```python
from build123d import *

# Parameters (mm, degrees)
SCHIZZO1_R                   = 14
ESTRUSIONE_ESTRUSIONE1_DEPTH = 40
SCHIZZO4_R                   = 2
TAGLIO_ESTRUSIONE1_DEPTH     = 10
SCHIZZO5_R                   = 2
TAGLIO_ESTRUSIONE2_DEPTH     = 10
SCHIZZO6_W                   = 32.003306677
SCHIZZO6_H                   = 7.880991961
TAGLIO_ESTRUSIONE3_DEPTH     = 20


with BuildPart() as part:
    # Schizzo1 → Estrusione-Estrusione1 (new body)
    with BuildSketch(Plane.XY):
        with BuildLine():
            Line((20, -13.266499161), (20, 13.266499161))
            ThreePointArc((20, 13.266499161), (0, 24), (-20, 13.266499161))
            Line((-20, 13.266499161), (-20, -13.266499161))
            ThreePointArc((-20, -13.266499161), (0, -24), (20, -13.266499161))
        make_face()
        Circle(SCHIZZO1_R, mode=Mode.SUBTRACT)
    extrude(amount=-ESTRUSIONE_ESTRUSIONE1_DEPTH)

    # Schizzo4 → Taglio-Estrusione1 (cut)
    with BuildSketch(Plane.ZY.offset(20)):
        with Locations((-10, 10)):
            Circle(SCHIZZO4_R)
        with Locations((-10, -10)):
            Circle(SCHIZZO4_R)
        with Locations((-30, -10)):
            Circle(SCHIZZO4_R)
        with Locations((-30, 10)):
            Circle(SCHIZZO4_R)
    extrude(amount=-TAGLIO_ESTRUSIONE1_DEPTH, mode=Mode.SUBTRACT)

    # Schizzo5 → Taglio-Estrusione2 (cut)
    with BuildSketch(Plane.XY):
        with Locations((-13.435028843, 13.435028843)):
            Circle(SCHIZZO5_R)
        with Locations((13.435028843, 13.435028843)):
            Circle(SCHIZZO5_R)
        with Locations((13.435028843, -13.435028843)):
            Circle(SCHIZZO5_R)
        with Locations((-13.435028843, -13.435028843)):
            Circle(SCHIZZO5_R)
    extrude(amount=-TAGLIO_ESTRUSIONE2_DEPTH, mode=Mode.SUBTRACT)

    # Schizzo6 → Taglio-Estrusione3 (cut)
    with BuildSketch(Plane(origin=(0, 0, -40), x_dir=(-1, 0, 0), z_dir=(0, 0, -1))):
        with Locations((0.127145472, 21.940495981)):
            Rectangle(SCHIZZO6_W, SCHIZZO6_H)
        with Locations((0.127145472, -21.940495981)):
            Rectangle(SCHIZZO6_W, SCHIZZO6_H)
    extrude(amount=-TAGLIO_ESTRUSIONE3_DEPTH, mode=Mode.SUBTRACT)


solid = part.part
```
Check sheet for the modelled part. Datum: model origin and axes. Units: mm. A direction names the side the tool comes from. Give positions to 0.01 mm unless a question says otherwise; leave off trailing zeros. Loops run counter-clockwise (first coordinate to the right, second up) from the corner with the lowest first, then second, coordinate; pieces in that order, holes last. Notation, with made-up numbers: M -11,-9.75 L 32,-9.75 A27 ccw 32,8.25 Z; hole C -17.75,49 d11. An arc over 180 degrees is marked long. Answer in a Markdown table with one row per item.
1) Cross-section at B-B (x = 0). Enter the section's corners in (y, z), plus the area to 3 significant figures.
Solutions:
| item | result |
|---|---|
| outline | M -24,-20 L -18,-20 L -18,-40 L -14,-40 L -14,0 L -24,0 Z; M 14,-40 L 18,-40 L 18,-20 L 24,-20 L 24,0 L 14,0 Z |
| area | 560 mm^2 |
2) Tool access check on faces 1 (the face through (0, 20, -20)), 2 (the face through (-15.1, -11.2, -11.6)), 3 (the face through (20, 0, -20)), 4 (the face through (0, 24, -15)), 5 (the face through (15.34, -12.83, -4.93)). Record the directions out of +Z, -Z, +X, -X, +Y, -Y that give a thin tool (end or side, any length) a straight path to the whole face; none if there is none.
Solutions:
| item | result |
|---|---|
| face 1 | -Z, +X, -X, +Y |
| face 2 | -X |
| face 3 | +Z, -Z, +X, +Y, -Y |
| face 4 | +Z, -Z, +Y |
| face 5 | +Z |
3) Depth check by flat-ended pin: pin 1 (3 mm diameter, centred on y = 16, z = -11, fed in from +X); pin 2 (0.7 mm diameter, centred on y = -11, z = -31, fed in from -X); pin 3 (3 mm diameter, centred on y = 18, z = -28.5, fed in from +X); pin 4 (10 mm diameter, centred on x = 5, z = -7.5, fed in from +Y). Enter the tip coordinate at first touch or a pass-through.
Solutions:
| item | result |
|---|---|
| pin 1 | stops at x = 19.12 |
| pin 2 | stops at x = -10 |
| pin 3 | stops at x = 17.43 |
| pin 4 | stops at y = 24 |
4) Cross-section at C-C (z = -37). Enter the section's corners in (x, y), plus the area to 3 significant figures.
Solutions:
| item | result |
|---|---|
| outline | M -20,-13.27 A24 ccw -15.87,-18 L 15.87,-18 A24 ccw 20,-13.27 L 20,13.27 A24 ccw 15.87,18 L -15.87,18 A24 ccw -20,13.27 Z; hole C 0,0 d28 |
| area | 789 mm^2 |
5) Cross-section at A-A (y = 0). Enter the section's corners in (x, z), plus the area to 3 significant figures.
Solutions:
| item | result |
|---|---|
| outline | M -20,-40 L -14,-40 L -14,0 L -20,0 Z; M 14,-40 L 20,-40 L 20,0 L 14,0 Z |
| area | 480 mm^2 |
6) Cross-section at D-D (x = 12.5). Enter the section's corners in (y, z).
Solutions:
| item | result |
|---|---|
| outline | M -20.49,-20 L -18,-20 L -18,-40 L -6.3,-40 L -6.3,0 L -11.67,0 L -11.67,-10 L -15.2,-10 L -15.2,0 L -20.49,0 Z; M 6.3,-40 L 18,-40 L 18,-20 L 20.49,-20 L 20.49,0 L 15.2,0 L 15.2,-10 L 11.67,-10 L 11.67,0 L 6.3,0 Z |
7) Thickness scan on line 1 (Z direction, x = -16.5, y = -10); line 2 (Y direction, x = -17, z = -30); line 3 (Y direction, x = -16, z = -10). Record the ranges inside material, lowest first.
Solutions:
| item | result |
|---|---|
| line 1 | z = -40 to -32, -28 to -12, -8 to 0 |
| line 2 | y = -16.94 to -12, -8 to 8, 12 to 16.94 |
| line 3 | y = -17.89 to -12, -8 to 8, 12 to 17.89 |
8) Mould release check, pull along X, two halves, no side actions. Record for faces 6 (the face through (-10, 11, -30)), 7 (the face through (-13.869, -15.387, -4.93)), 8 (the face through (13, -13, -10)), 9 (the face through (0, -18, -30)): released by +X, released by -X, zero draft, split by the parting line, or undercut.
Solutions:
| item | result |
|---|---|
| face 6 | released by -X |
| face 7 | undercut |
| face 8 | undercut |
| face 9 | zero draft |
